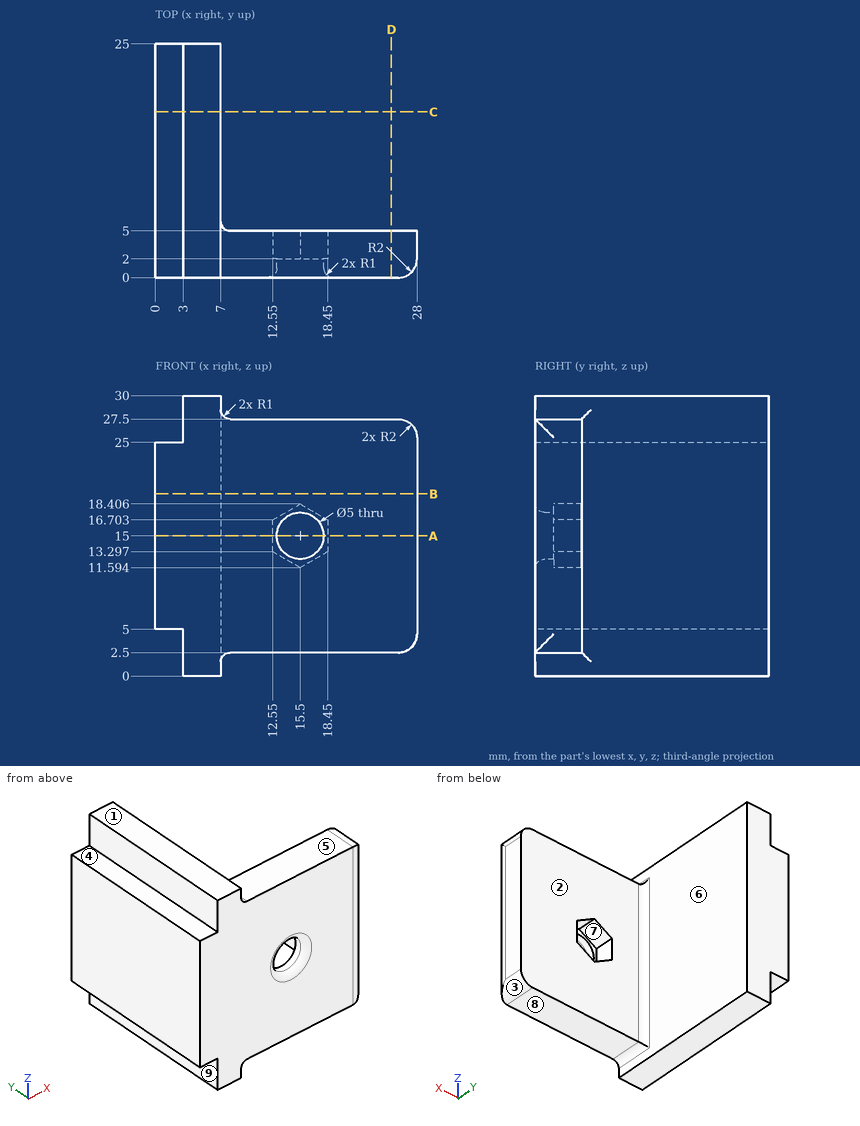
Can you work these out from the drawing? Everything is in mm from the part's minimum corner. A direction names the side the tool comes from. Give positions to 0.01 mm unless a question says otherwise; leave off trailing zeros. Loops run counter-clockwise (first coordinate to the right, second up) from the corner with the lowest first, then second, coordinate; pieces in that order, holes last. Notation, with made-up numbers: (-10.5, 17.5) -> (12.5, 17.5) arc R21 cw to (12.5, 50.5) -> close; hole circle Ø10 at (-11.75, 39). An arc over 180 degrees is marked (long way). Put each result on its own line as item: value.
(1) For the marked faces 1, 2, 3, 4 and 5, which set-ups out of +Z, -Z, +X, -X, +Y, -Y let a thin tool reach every point of the face, with its end or its side?
Computed:
face 1: +Z, +X, -X, +Y, -Y
face 2: +Z, -Z, +X, +Y
face 3: -Z, +X, +Y, -Y
face 4: +Z, -X, +Y, -Y
face 5: +Z, +X, +Y, -Y
(2) Thinking about a two-plate mould opening in X: for the marked faces 6, 7, 8 and 9, which applies, pulls with the +X half, pulls with the -X half, needs draft (parallel to the pull), parting line crosses it, or undercut?
Computed:
face 6: pulls with the +X half
face 7: undercut
face 8: needs draft
face 9: pulls with the -X half
(3) Imagine slicing it at D-D on x = 25.25. Write out the boundary of the cut face in (y, z).
Computed:
outline: (0, 2.5) -> (5, 2.5) -> (5, 27.5) -> (0, 27.5) -> close
(4) Imagine slicing it at A-A on z = 15. Write out the boundary of the cut face in (x, y).
Computed:
outline: (0, 0) -> (12, 0) arc R1 ccw to (13, 1) -> (13, 2) -> (12.55, 2) -> (12.55, 5) -> (8, 5) arc R1 cw to (7, 6) -> (7, 25) -> (0, 25) -> close; (18, 1) arc R1 ccw to (19, 0) -> (26, 0) arc R2 ccw to (28, 2) -> (28, 5) -> (18.45, 5) -> (18.45, 2) -> (18, 2) -> close
(5) Imagine slicing it at C-C on y = 17.75. Write out the boundary of the cut face in (x, z).
Computed:
outline: (0, 5) -> (3, 5) -> (3, 0) -> (7, 0) -> (7, 30) -> (3, 30) -> (3, 25) -> (0, 25) -> close
(6) Please list where these lines run through material, in increasing order: probe 1 along Z at (x, y) = (15.5, 1.75); probe 2 along X at (y, z) = (10.5, 28); probe 3 along Z at (x, y) = (21, 1.75). Write a range as [from, to].
Computed:
probe 1: [2.5, 12.5], [17.5, 27.5]
probe 2: [3, 7]
probe 3: [2.5, 27.5]
(7) Imagine slicing it at B-B on z = 19.5. Write out the boundary of the cut face in (x, y), plus the area to 3 significant figures.
Computed:
outline: (0, 0) -> (26, 0) arc R2 ccw to (28, 2) -> (28, 5) -> (8, 5) arc R1 cw to (7, 6) -> (7, 25) -> (0, 25) -> close
area: 279 mm^2
(8) I'm going to push flat-ended pins straight in: pin 1 Ø8 at (x, z) = (15.5, 15) entering from +Y; pin 2 Ø7.5 at (y, z) = (14.5, 21.5) entering from +X; pin 3 Ø0.9 at (x, y) = (1, 18) entering from +Z. Where does each tip first touch, or does it pass through?
Computed:
pin 1: y = 5
pin 2: x = 7
pin 3: z = 25
